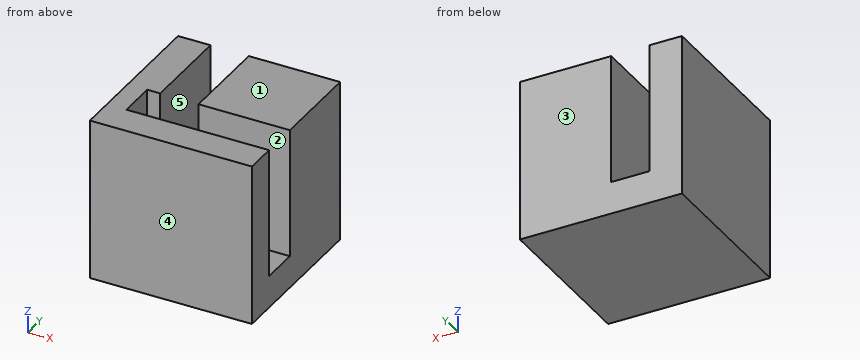
```python
from build123d import *

# Parameters (mm, degrees)
F0_W     = 7.16
F0_H     = 7.2381474632
F1_DEPTH = 10.16
F2_W     = 7.16
F2_H     = 7.2381474632
F3_DEPTH = 2.54


with BuildPart() as f1:
    # F0 (on Top) → F1 (new body)
    with BuildSketch(Plane.XY):
        with Locations((-5.8439813066, -2.7033329925)):
            Rectangle(F0_W, F0_H)
    extrude(amount=F1_DEPTH)



with BuildPart() as f1b:
    # F0 (on Top) → F1, piece 2 (new body)
    with BuildSketch(Plane.XY):
        Polygon((-12.4239813066, 0.9157407391), (-14.9639813066, 0.9157407391), (-14.9639813066, -11.7842592609), (-2.2639813066, -11.7842592609), (-2.2639813066, -9.3224067241), (-9.4239813066, -9.3224067241), (-12.4239813066, -9.3224067241), (-13.4399813066, -9.3224067241), (-13.4399813066, -6.3224067241), (-12.4239813066, -6.3224067241), align=None)
    extrude(amount=F1_DEPTH)


with BuildPart() as f1_1:
    add(f1.part)

    add(f1b.part)  # F3 merges F1b
    # F2 (on face) → F3 (join)
    with BuildSketch(Plane(origin=(0, 0, 0), x_dir=(1, 0, 0), z_dir=(0, 0, -1))):
        with Locations((-5.8439813066, 2.7033329925)):
            Rectangle(F2_W, F2_H)
        Polygon((-2.2639813066, 9.3224067241), (-13.4399813066, 9.3224067241), (-13.4399813066, 6.3224067241), (-12.4239813066, 6.3224067241), (-12.4239813066, -0.9157407391), (-9.4239813066, -0.9157407391), (-9.4239813066, 6.3224067241), (-2.2639813066, 6.3224067241), align=None)
        Polygon((-13.4399813066, 6.3224067241), (-13.4399813066, 9.3224067241), (-2.2639813066, 9.3224067241), (-2.2639813066, 11.7842592609), (-14.9639813066, 11.7842592609), (-14.9639813066, -0.9157407391), (-12.4239813066, -0.9157407391), (-12.4239813066, 6.3224067241), align=None)
    extrude(amount=F3_DEPTH)


solid = f1_1.part
```
CAD build for the part. Positions are in the model's coordinates, mm. Face numbers are marked on the shaded views. A direction names the side the tool comes from. Round coordinates to 2 decimals unless told otherwise and drop trailing zeros. Order: outer loops, then holes, each group sorted by start corner. A loop starts at its lowest first (then second) coordinate and runs counter-clockwise, first axis right, second up. Notation, with made-up numbers: (88, 10) - (119, 10) arc R19 cw to (119, 38) - close; hole circle Ø7 at (0.5, -36.5). An arc over 180 degrees is marked (long way). Answer as CSV lines item,"result". Start each with the question number.
1. Saw through at D-D, the plane y = -7.75. Write the cut outline in (x, z), and give its area (3 significant figures).
2. Pull direction Y, two halves, no side cores. Call the marked faces 1, 2 and 3: +Y half, -Y half, draft (parallel to the pull), parting line (faces both ways), or undercut.
3. Drill centre lines: L1, parallel to X at y = -0.75, z = 2.25; L2, parallel to Y at x = -7.5, z = 5.25; L3, parallel to Y at x = -10.5, z = 3.25. Where is each one in solid material? Low to high. Write a range as [from, to].
4. Saw through at B-B, the plane y = -5. Write the cut outline in (x, z), and give its area (3 significant figures).
5. Tool access for the marked faces 4 and 5: list every direction of +Z, -Z, +X, -X, +Y, -Y with a clear straight run to the whole face (end or side of a thin tool).
6. Saw through at C-C, the plane x = -7.5. Write the cut outline in (y, z).
7. Saw through at A-A, the plane z = 5.75. Write the cut outline in (x, y).
Model answer:
1,outline,"(-14.96, -2.54) - (-2.26, -2.54) - (-2.26, 0) - (-13.44, 0) - (-13.44, 10.16) - (-14.96, 10.16) - close"
1,area,"47.7 mm²"
2,face 1,"draft"
2,face 2,"undercut"
2,face 3,"+Y half"
3,L1,"x = [-14.96, -12.42], [-9.42, -2.26]"
3,L2,"y = [-11.78, -9.32], [-6.32, 0.92]"
3,L3,"y = [-11.78, -9.32]"
4,outline,"(-14.96, -2.54) - (-2.26, -2.54) - (-2.26, 10.16) - (-9.42, 10.16) - (-9.42, 0) - (-12.42, 0) - (-12.42, 10.16) - (-14.96, 10.16) - close"
4,area,"131 mm²"
5,face 4,"+Z, -Z, +X, -X, -Y"
5,face 5,"+Z, +Y"
6,outline,"(-11.78, -2.54) - (0.92, -2.54) - (0.92, 10.16) - (-6.32, 10.16) - (-6.32, 0) - (-9.32, 0) - (-9.32, 10.16) - (-11.78, 10.16) - close"
7,outline,"(-14.96, -11.78) - (-2.26, -11.78) - (-2.26, -9.32) - (-13.44, -9.32) - (-13.44, -6.32) - (-12.42, -6.32) - (-12.42, 0.92) - (-14.96, 0.92) - close; (-9.42, -6.32) - (-2.26, -6.32) - (-2.26, 0.92) - (-9.42, 0.92) - close"
